Geometry: final body of the model. Coordinates: model frame, mm. A direction names the side the tool comes from. Coordinates: 2 decimals unless noted, no trailing zeros. Loops run counter-clockwise (first coordinate to the right, second up) from the corner with the lowest first, then second, coordinate; pieces in that order, holes last. Notation, with made-up numbers: (-10.5, -6) - (30.5, -6) arc R12 ccw to (30.5, 0) - close; hole circle Ø11 at (-38.75, 1.25). An arc over 180 degrees is marked (long way). Return JSON: item names as keys, results as strings.
from build123d import *

# Parameters (mm, degrees)
F0_R     = 2.75
F1_DEPTH = 3
F2_R     = 2.75
F3_DEPTH = 2.65684
F4_R     = 1
F5_R     = 2
F6_R     = 10


with BuildPart() as f1:
    # F0 (on Front) → F1 (new body)
    with BuildSketch(Plane.XZ):
        Polygon((-10.85, 10), (-60, 10), (-60, -10), (-10.85, -10), (0, -11.7585089141), (0, 8.2414910859), align=None)
        with Locations((-50, 0)):
            Circle(F0_R, mode=Mode.SUBTRACT)
        with BuildLine():
            ThreePointArc((-27.1, -2.75), (-29.85, 0), (-27.1, 2.75))
            Line((-27.1, 2.75), (-24.6, 2.75))
            ThreePointArc((-24.6, 2.75), (-21.85, 0), (-24.6, -2.75))
            Line((-24.6, -2.75), (-27.1, -2.75))
        make_face(mode=Mode.SUBTRACT)
        Polygon((20, 5), (0, 8.2414910859), (0, -11.7585089141), (20, -15), (40, -15), (40, -8.5), (34, -8.5), (34, -1.5), (40, -1.5), (40, 5), align=None)
        with Locations((30, -5)):
            Circle(F0_R, mode=Mode.SUBTRACT)
    extrude(amount=F1_DEPTH)

    # F2 (on face) → F3 (join)
    with BuildSketch(Plane.XZ.offset(3)):
        Polygon((20, -15), (40, -15), (40, -8.5), (34, -8.5), (34, -1.5), (40, -1.5), (40, 5), (20, 5), align=None)
        with Locations((30, -5)):
            Circle(F2_R, mode=Mode.SUBTRACT)
        Polygon((0, -11.7585089141), (20, -15), (20, 5), (0, 8.2414910859), align=None)
    extrude(amount=F3_DEPTH)

    # F4
    f4_edges = [f1.edges().sort_by_distance(p)[0] for p in [
        (34, -2.82842, -1.5),
        (34, -2.82842, -8.5),
    ]]
    fillet(f4_edges, radius=F4_R)

    # F5
    f5_edges = [f1.edges().sort_by_distance(p)[0] for p in [
        (40, -2.82842, 5),
        (40, -2.82842, -8.5),
        (40, -2.82842, -1.5),
        (40, -2.82842, -15),
        (-60, -1.5, 10),
        (-60, -1.5, -10),
    ]]
    fillet(f5_edges, radius=F5_R)

    # F6
    f6_edges = [f1.edges().sort_by_distance(p)[0] for p in [
        (-10.85, -1.5, 10),
        (20, -2.82842, 5),
        (-10.85, -1.5, -10),
        (20, -2.82842, -15),
    ]]
    fillet(f6_edges, radius=F6_R)


solid = f1.part
Item 1: Ray query, probe 1 along Z at (x, y) = (30, -2.4); probe 2 along Z at (x, y) = (-50, -1.15); probe 3 along Y at (x, z) = (-37.5, 3.5). Return the intervals inside material, ascending. Write a range as from..to.
Worked out:
{"probe 1": "-15..-7.75, -2.25..5", "probe 2": "-10..-2.75, 2.75..10", "probe 3": "-3..0"}
Item 2: Section query D-D, the plane x = 30. Return loops of the section in (y, z), and give its area (3 significant figures).
Worked out:
{"outline": "(-5.66, -15) - (0, -15) - (0, -7.75) - (-5.66, -7.75) - close; (-5.66, -2.25) - (0, -2.25) - (0, 5) - (-5.66, 5) - close", "area": "82.0 mm^2"}
Item 3: Mould query, pull axis Z, two halves, no side actions, for faces 1 (the face through (-30, -3, -1)), 2 (the face through (8.03, -2.79, 6.94)), 3 (the face through (-26, -1, -2.75)). Classes: +Z half, -Z half, draft (parallel to the pull), parting line (faces both ways), or undercut.
Worked out:
{"face 1": "draft", "face 2": "+Z half", "face 3": "undercut"}
Item 4: Section query B-B, the plane z = -5. Return loops of the section in (x, y).
Worked out:
{"outline": "(-60, -3) - (0, -3) - (0, -5.66) - (27.25, -5.66) - (27.25, 0) - (-60, 0) - close; (32.75, -5.66) - (34, -5.66) - (34, 0) - (32.75, 0) - close"}
Item 5: First-contact query: pin 1 Ø6 at (x, z) = (-7, -5.5) entering from -Y; pin 2 Ø3 at (x, y) = (-5.5, -2) entering from -Z; pin 3 Ø1.3 at (y, z) = (-4, -2.5) entering from -X. Flat tips, straight axial feed; report the tip coordinate or a pass-through.
Worked out:
{"pin 1": "y = -3", "pin 2": "z = -11.11", "pin 3": "x = 0"}
Item 6: Reachability of faces 4 (the face through (-10.841, -1.521, -10.033)), 5 (the face through (-29.85, -1.48, -0.06)), 6 (the face through (34, -3, -5)) from +Z, -Z, +X, -X, +Y, -Y: full face, straight path, thin tool, end or side. Return the list, or none.
Worked out:
{"face 4": "-Z, -X, +Y, -Y", "face 5": "+Y, -Y", "face 6": "+X, +Y, -Y"}
Item 7: Section query C-C, the plane y = -1.35. Count the separate pieces of the cut face and the enclosed holes in it, and give its area (3 significant figures).
Worked out:
{"separate pieces": "1", "enclosed holes": "3", "area": "1,870 mm^2"}
Item 8: Section query A-A, the plane x = -50. Return loops of the section in (y, z), and give its area (3 significant figures).
Worked out:
{"outline": "(-3, -10) - (0, -10) - (0, -2.75) - (-3, -2.75) - close; (-3, 2.75) - (0, 2.75) - (0, 10) - (-3, 10) - close", "area": "43.5 mm^2"}
